CAD build for the part. Positions are in the model's coordinates, mm. Face numbers are marked on the shaded views. A direction names the side the tool comes from. Coordinates: 2 decimals unless noted, no trailing zeros. Order: outer loops, then holes, each group sorted by start corner. A loop starts at its lowest first (then second) coordinate and runs counter-clockwise, first axis right, second up. Notation, with made-up numbers: (83.25, 81.5) - (100.25, 81.5) arc R17 cw to (100.25, 113.5) - close; hole circle Ø5 at (-31, 28). An arc over 180 degrees is marked (long way). Write each question's results on one line, items separated by ' | '. Start each with the question number.
Q1. Wall check: probe 1 along X at (y, z) = (-6.25, 0); probe 2 along Y at (x, z) = (-6, 1.75); probe 3 along X at (y, z) = (12, 0.25). Give the ranges that are in metal, low to high.
Q2. Band-saw the part on C-C, the plane y = 17.5. Write the cut outline in (x, z), then the cut area to 3 significant figures.
Q3. Which spindle directions (+Z, -Z, +X, -X, +Y, -Y) get a long thin tool onto all of the face, cutting with end or side? Do the marked faces 1, 2, 3 and 4. Say none if no direction does.
Q4. Pull direction X, two halves, no side cores. Call the marked faces 5, 6 and 7: released by +X, released by -X, zero draft, split by the parting line, or undercut.
Q5. Pin check, flat tips, straight feed: P1, Ø10.5, axis at x = -5, y = 13, coming from the +Z side; P2, Ø6, axis at x = -15, z = 9.5, coming from the +Y side; P3, Ø2, axis at x = -15, z = 0, coming from the -Y side. Stop position of each tip, or through.
Q6. Band-saw the part on B-B, the plane x = 6. Write the cut outline in (y, z).
Q7. Band-saw the part on A-A, the plane y = 0. Write the cut outline in (x, z).
Q8. Band-saw the part on D-D, the plane z = 0. Count the separate pieces of the cut face and the enclosed holes in it, then the cut area to 3 significant figures.
```python
from build123d import *

# Parameters (mm, degrees)
SKETCH_1_W             = 35
SKETCH_1_H             = 50
SKETCH_1_W_2           = 16
SKETCH_1_H_2           = 8.4
EXTRUDE_564_DEPTH      = 5
SKETCH_2_W             = 5.75
SKETCH_2_H             = 8.4
CUT_EXTRUDE_879_DEPTH  = 8.5
FILLET_1_R             = 1
SKETCH_3_R             = 1.25
CUT_EXTRUDE_1403_DEPTH = 8
SKETCH_10_R            = 1.25
CUT_EXTRUDE_1593_DEPTH = 10
SKETCH_11_W            = 20
SKETCH_11_H            = 26.5
CUT_EXTRUDE_1977_DEPTH = 42.432957896
FILLET_2_R             = 3
SKETCH_13_W            = 5
SKETCH_13_H            = 8
EXTRUDE_4716_DEPTH     = 9.6
SKETCH_16_W            = 5
SKETCH_16_H            = 7
EXTRUDE_5207_DEPTH     = 0.4
SKETCH_14_R            = 1.25
CUT_EXTRUDE_5724_DEPTH = 46.55491192
FILLET_3_R             = 3
FILLET_4_R             = 1
FILLET_5_R             = 1
CUT_EXTRUDE_6952_REACH = 43.433
SKETCH_17_W            = 19
SKETCH_17_H            = 5
FILLET_6_R             = 2.5
FILLET_7_R             = 1


# Some blends are built 0.0001 mm under size
with BuildPart() as part:
    # Эскиз1 → Extrude 564 (new, symmetric)
    with BuildSketch(Plane.XY):
        with Locations((0, 11.2)):
            Rectangle(SKETCH_1_W, SKETCH_1_H)
        Rectangle(SKETCH_1_W_2, SKETCH_1_H_2, mode=Mode.SUBTRACT)
    extrude(amount=EXTRUDE_564_DEPTH, both=True)

    # Эскиз2 → Cut-Extrude 879 (cut)
    with BuildSketch(Plane.XY.offset(5)):
        with Locations((-10.875, 0)):
            Rectangle(SKETCH_2_W, SKETCH_2_H)
        with Locations((10.875, 0)):
            Rectangle(SKETCH_2_W, SKETCH_2_H)
    extrude(amount=-CUT_EXTRUDE_879_DEPTH, mode=Mode.SUBTRACT)

    # Скругление1
    fillet_1_edges = [part.edges().sort_by_distance(p)[0] for p in [
        (-13.75, -4.2, 0.75),
        (-13.75, 4.2, 0.75),
        (13.75, 4.2, 0.75),
        (13.75, -4.2, 0.75),
    ]]
    fillet(fillet_1_edges, radius=FILLET_1_R)

    # Эскиз3 → Cut-Extrude 1403 (cut)
    with BuildSketch(Plane.XY.offset(-3.5)):
        with Locations((-10.3, 0)):
            Circle(SKETCH_3_R)
        with Locations((10.3, 0)):
            Circle(SKETCH_3_R)
    extrude(amount=-CUT_EXTRUDE_1403_DEPTH, mode=Mode.SUBTRACT)

    # Эскиз10 → Cut-Extrude 1593 (cut)
    with BuildSketch(Plane.XZ.offset(13.8)):
        with Locations(Location((-15, 0, 0), (0, 0, 270))):
            Circle(SKETCH_10_R)
        with Locations(Location((15, 0, 0), (0, 0, 270))):
            Circle(SKETCH_10_R)
    cut_extrude_1593 = extrude(amount=-CUT_EXTRUDE_1593_DEPTH, mode=Mode.SUBTRACT)

    # Mirror 1655: Cut-Extrude 1593 across plane
    add(cut_extrude_1593.mirror(Plane.ZX.offset(11.2)), mode=Mode.SUBTRACT)

    # Эскиз11 → Cut-Extrude 1977 (cut, through all)
    with BuildSketch(Plane.XY.offset(5)):
        with Locations((0, 20.45)):
            Rectangle(SKETCH_11_W, SKETCH_11_H)
    extrude(amount=-CUT_EXTRUDE_1977_DEPTH, mode=Mode.SUBTRACT)

    # Скругление2
    fillet_2_edges = [part.edges().sort_by_distance(p)[0] for p in [
        (10, 7.2, 0),
        (-10, 7.2, 0),
        (-10, 33.7, 0),
        (10, 33.7, 0),
    ]]
    fillet(fillet_2_edges, radius=FILLET_2_R)

    # Эскиз13 → Extrude 4716 (add)
    with BuildSketch(Plane.XZ.offset(13.8)):
        with Locations((-15, 9)):
            Rectangle(SKETCH_13_W, SKETCH_13_H)
        with Locations((15, 9)):
            Rectangle(SKETCH_13_W, SKETCH_13_H)
    extrude(amount=-EXTRUDE_4716_DEPTH)

    # Эскиз16 → Extrude 5207 (add)
    with BuildSketch(Plane(origin=(0, -4.2, 0), x_dir=(1, 0, 0), z_dir=(0, 1, 0))):
        with Locations((-15, -9.5)):
            Rectangle(SKETCH_16_W, SKETCH_16_H)
        with Locations((15, -9.5)):
            Rectangle(SKETCH_16_W, SKETCH_16_H)
    extrude(amount=EXTRUDE_5207_DEPTH)

    # Эскиз14 → Cut-Extrude 5724 (cut, through all)
    with BuildSketch(Plane(origin=(0, -3.8, 0), x_dir=(1, 0, 0), z_dir=(0, 1, 0))):
        with Locations(Location((-15, -10, 0), (0, 0, 270))):
            Circle(SKETCH_14_R)
        with Locations(Location((15, -10, 0), (0, 0, 90))):
            Circle(SKETCH_14_R)
    extrude(amount=-CUT_EXTRUDE_5724_DEPTH, mode=Mode.SUBTRACT)

    # Скругление3
    # the kernel refuses this fillet: 3 mm, written as the material it adds along each edge
    with BuildSketch(Plane(origin=(12.5, -13.8, 5), x_dir=(-1, 0, 0), z_dir=(0, 1, 0))) as fillet_3_piece_1_section:
        with BuildLine():
            CenterArc((FILLET_3_R, FILLET_3_R), FILLET_3_R, 180, 90)
            Line((0, FILLET_3_R), (0, 0))
            Line((0, 0), (FILLET_3_R, 0))
        make_face()
    fillet_3_piece_1 = extrude(amount=9.6, mode=Mode.PRIVATE)
    fillet_3_piece_1 = split(fillet_3_piece_1, bisect_by=Plane(origin=(11.641402177, -9, 6), z_dir=(0, 0, -1)), keep=Keep.TOP, mode=Mode.PRIVATE)
    add(fillet_3_piece_1)
    with BuildSketch(Plane(origin=(12.5, -13.8, 5), x_dir=(-1, 0, 0), z_dir=(0, 1, 0))) as fillet_3_piece_2_section:
        with BuildLine():
            CenterArc((FILLET_3_R, FILLET_3_R), FILLET_3_R, 180, 90)
            Line((0, FILLET_3_R), (0, 0))
            Line((0, 0), (FILLET_3_R, 0))
        make_face()
    fillet_3_piece_2 = extrude(amount=9.6, mode=Mode.PRIVATE)
    fillet_3_piece_2 = split(fillet_3_piece_2, bisect_by=Plane(origin=(12.327479681, -9, 6), z_dir=(0, 0, 1)), keep=Keep.TOP, mode=Mode.PRIVATE)
    add(fillet_3_piece_2)
    with BuildSketch(Plane(origin=(12.5, -13.8, 5), x_dir=(-1, 0, 0), z_dir=(0, 1, 0))) as fillet_3_piece_3_section:
        with BuildLine():
            CenterArc((FILLET_3_R, FILLET_3_R), FILLET_3_R, 180, 90)
            Line((0, FILLET_3_R), (0, 0))
            Line((0, 0), (FILLET_3_R, 0))
        make_face()
    fillet_3_piece_3 = extrude(amount=17.1, mode=Mode.PRIVATE)
    fillet_3_piece_3 = split(fillet_3_piece_3, bisect_by=Plane(origin=(12.327479681, -4.2, 6.589070595), z_dir=(0, 1, 0)), keep=Keep.TOP, mode=Mode.PRIVATE)
    fillet_3_piece_3 = split(fillet_3_piece_3, bisect_by=Plane(origin=(12.327479681, -3.8, 6.589070595), z_dir=(0, -1, 0)), keep=Keep.TOP, mode=Mode.PRIVATE)
    fillet_3_piece_3 = split(fillet_3_piece_3, bisect_by=Plane(origin=(12.327479681, -4, 6), z_dir=(0, 0, 1)), keep=Keep.TOP, mode=Mode.PRIVATE)
    add(fillet_3_piece_3)
    with BuildSketch(Plane(origin=(-12.5, -13.8, 5), x_dir=(0, 0, 1), z_dir=(0, 1, 0))) as fillet_3_piece_4_section:
        with BuildLine():
            CenterArc((FILLET_3_R, FILLET_3_R), FILLET_3_R, 180, 90)
            Line((0, FILLET_3_R), (0, 0))
            Line((0, 0), (FILLET_3_R, 0))
        make_face()
    fillet_3_piece_4 = extrude(amount=9.6, mode=Mode.PRIVATE)
    fillet_3_piece_4 = split(fillet_3_piece_4, bisect_by=Plane(origin=(-12.327479681, -9, 6), z_dir=(0, 0, 1)), keep=Keep.TOP, mode=Mode.PRIVATE)
    add(fillet_3_piece_4)
    with BuildSketch(Plane(origin=(-12.5, -13.8, 5), x_dir=(0, 0, 1), z_dir=(0, 1, 0))) as fillet_3_piece_5_section:
        with BuildLine():
            CenterArc((FILLET_3_R, FILLET_3_R), FILLET_3_R, 180, 90)
            Line((0, FILLET_3_R), (0, 0))
            Line((0, 0), (FILLET_3_R, 0))
        make_face()
    fillet_3_piece_5 = extrude(amount=9.6, mode=Mode.PRIVATE)
    fillet_3_piece_5 = split(fillet_3_piece_5, bisect_by=Plane(origin=(-11.641402177, -9, 6), z_dir=(0, 0, -1)), keep=Keep.TOP, mode=Mode.PRIVATE)
    add(fillet_3_piece_5)
    with BuildSketch(Plane(origin=(-12.5, -13.8, 5), x_dir=(0, 0, 1), z_dir=(0, 1, 0))) as fillet_3_piece_6_section:
        with BuildLine():
            CenterArc((FILLET_3_R, FILLET_3_R), FILLET_3_R, 180, 90)
            Line((0, FILLET_3_R), (0, 0))
            Line((0, 0), (FILLET_3_R, 0))
        make_face()
    fillet_3_piece_6 = extrude(amount=17.1, mode=Mode.PRIVATE)
    fillet_3_piece_6 = split(fillet_3_piece_6, bisect_by=Plane(origin=(-12.327479681, -4.2, 6.589070595), z_dir=(0, 1, 0)), keep=Keep.TOP, mode=Mode.PRIVATE)
    fillet_3_piece_6 = split(fillet_3_piece_6, bisect_by=Plane(origin=(-12.327479681, -4, 6), z_dir=(0, 0, 1)), keep=Keep.TOP, mode=Mode.PRIVATE)
    fillet_3_piece_6 = split(fillet_3_piece_6, bisect_by=Plane(origin=(-12.327479681, -3.8, 6.589070595), z_dir=(0, -1, 0)), keep=Keep.TOP, mode=Mode.PRIVATE)
    add(fillet_3_piece_6)
    # the kernel refuses this fillet: 3 mm, written as the material it takes off along each edge
    with BuildSketch(Plane(origin=(17.5, 3.7, 13), x_dir=(-1, 0, 0), z_dir=(0, -1, 0)), Plane(origin=(12.5, -21.3, 13), x_dir=(1, 0, 0), z_dir=(0, 1, 0)), Plane(origin=(-17.5, -21.3, 13), x_dir=(1, 0, 0), z_dir=(0, 1, 0)), Plane(origin=(-12.5, -21.3, 13), x_dir=(0, 0, -1), z_dir=(0, 1, 0))) as fillet_3_2_piece_1:
        with BuildLine():
            CenterArc((FILLET_3_R, FILLET_3_R), FILLET_3_R, 180, 90)
            Line((0, FILLET_3_R), (0, 0))
            Line((0, 0), (FILLET_3_R, 0))
        make_face()
    extrude(amount=25, mode=Mode.SUBTRACT)

    # Скругление4
    fillet_4_edges = [part.edges().sort_by_distance(p)[0] for p in [
        (15.125, -4.2, 5),
        (-15.125, -4.2, 5),
    ]]
    fillet(fillet_4_edges, radius=FILLET_4_R - 0.0001)  # a hair under: the kernel refuses the full size

    # Скругление5
    # the kernel refuses this fillet: 1 mm, written as the material it takes off along each edge
    with BuildSketch(Plane(origin=(9.736067977, -3.8, 6), x_dir=(0, 0, 1), z_dir=(1, 0, 0))) as fillet_5_piece_1:
        with BuildLine():
            CenterArc((0.8, 1), FILLET_5_R, 216.869897646, 53.130102354)
            Line((0, 0.4), (-0.016, 0.388))
            ThreePointArc((-0.016, 0.388), (-0.02, 0.2), (-0.02, 0))
            Line((-0.02, 0), (0, -0.02))
            Line((0, -0.02), (0.8, -0.02))
            Line((0.8, -0.02), (0.8, 0))
        make_face()
    extrude(amount=9.763932023, mode=Mode.SUBTRACT)
    with BuildSketch(Plane(origin=(-9.736067977, -3.8, 6), x_dir=(0, -1, 0), z_dir=(-1, 0, 0))) as fillet_5_piece_2:
        with BuildLine():
            CenterArc((1, 0.8), FILLET_5_R, 180, 53.130102354)
            Line((0, 0.8), (-0.02, 0.8))
            Line((-0.02, 0.8), (-0.02, 0))
            Line((-0.02, 0), (0, -0.02))
            ThreePointArc((0, -0.02), (0.2, -0.02), (0.388, -0.016))
            Line((0.388, -0.016), (0.4, 0))
        make_face()
    extrude(amount=9.763932023, mode=Mode.SUBTRACT)

    # Эскиз17 → Cut-Extrude 6952 (cut, up to next)
    with BuildSketch(Plane.XY.offset(5), mode=Mode.PRIVATE) as cut_extrude_6952_sk1:
        with Locations((0, -9)):
            Rectangle(SKETCH_17_W, SKETCH_17_H)
    cut_extrude_6952_tool1 = extrude(cut_extrude_6952_sk1.sketch, amount=-CUT_EXTRUDE_6952_REACH, mode=Mode.PRIVATE) & part.part
    add(cut_extrude_6952_tool1.solids().sort_by_distance((0, -9, 5))[0], mode=Mode.SUBTRACT)

    # Скругление6
    fillet_6_edges = [part.edges().sort_by_distance(p)[0] for p in [
        (9.5, -6.5, 0),
        (9.5, -11.5, 0),
        (-9.5, -6.5, 0),
        (-9.5, -11.5, 0),
    ]]
    fillet(fillet_6_edges, radius=FILLET_6_R - 0.0001)  # a hair under: the kernel refuses the full size

    # Скругление7
    fillet_7_edges = [part.edges().sort_by_distance(p)[0] for p in [
        (0, -6.5, -5),
        (0, -6.5, 5),
        (0, -11.5, -5),
        (0, -11.5, 5),
        (8.767796242, -7.232203758, 5),
        (8.767796242, -7.232203758, -5),
        (8.767796242, -10.767796242, 5),
        (8.767796242, -10.767796242, -5),
        (-8.767796242, -7.232203758, 5),
        (-8.767796242, -7.232203758, -5),
        (-8.767796242, -10.767796242, 5),
        (-8.767796242, -10.767796242, -5),
    ]]
    fillet(fillet_7_edges, radius=FILLET_7_R)


solid = part.part
```
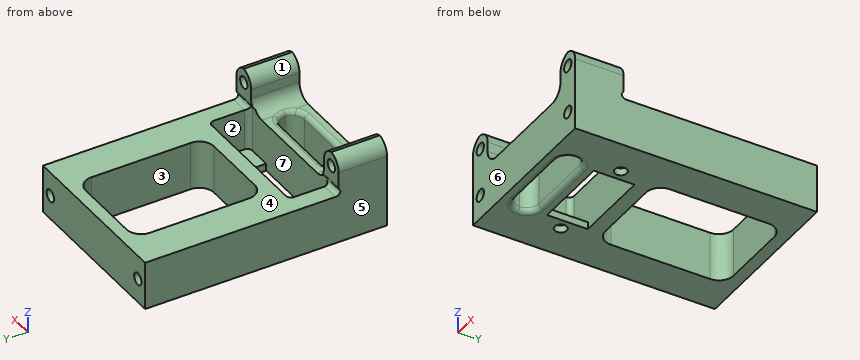
Results below:
1) probe 1: x = -17.5 to -16.25, -13.75 to 13.75, 16.25 to 17.5 | probe 2: y = -13.8 to -11.5, -6.5 to -4.2, 4.2 to 7.2, 33.7 to 36.2 | probe 3: x = -17.5 to -10, 10 to 17.5
2) outline: (-17.5, -5) - (-10, -5) - (-10, 5) - (-17.5, 5) - close; (10, -5) - (17.5, -5) - (17.5, 5) - (10, 5) - close | area: 150 mm²
3) face 1: +Z, +Y, -Y | face 2: +Z | face 3: +Z, -Z | face 4: +Z, +X, -X, +Y
4) face 5: released by -X | face 6: zero draft | face 7: undercut
5) P1: stops at z = 5 | P2: stops at y = -3.8 | P3: stops at y = -3.8
6) outline: (-13.8, -5) - (-12.5, -5) arc R1 ccw to (-11.5, -4) - (-11.5, 4) arc R1 ccw to (-12.5, 5) - (-13.8, 5) - close; (-6.5, -4) arc R1 ccw to (-5.5, -5) - (-4.2, -5) - (-4.2, 5) - (-5.5, 5) arc R1 ccw to (-6.5, 4) - close; (4.2, -5) - (7.2, -5) - (7.2, 5) - (4.2, 5) - close; (33.7, -5) - (36.2, -5) - (36.2, 5) - (33.7, 5) - close
7) outline: (-17.5, -5) - (-11.55, -5) - (-11.55, -3.5) - (-13.75, -3.5) - (-13.75, 5) - (-17.5, 5) - close; (-9.05, -5) - (-8, -5) - (-8, -3.5) - (-9.05, -3.5) - close; (8, -5) - (9.05, -5) - (9.05, -3.5) - (8, -3.5) - close; (11.55, -5) - (17.5, -5) - (17.5, 5) - (13.75, 5) - (13.75, -3.5) - (11.55, -3.5) - close
8) separate pieces: 1 | enclosed holes: 3 | area: 808 mm²
